```python
from build123d import *

# Parameters (mm, degrees)
SKETCH1_W           = 174
SKETCH1_H           = 148
SKETCH1_R           = 66
SKETCH1_R_2         = 2.15
BOSS_EXTRUDE1_DEPTH = 5
FILLET1_R           = 40


with BuildPart() as part:
    # Sketch1 → Boss-Extrude1 (new body)
    with BuildSketch(Plane(origin=(0, 0, 0), x_dir=(1, 0, 0), z_dir=(0, 1, 0))):
        Rectangle(SKETCH1_W, SKETCH1_H)
        with Locations(Location((0, 0, 0), (0, 0, 270))):
            Circle(SKETCH1_R, mode=Mode.SUBTRACT)
        with Locations(Location((75, 36, 0), (0, 0, 270))):
            Circle(SKETCH1_R_2, mode=Mode.SUBTRACT)
        with Locations(Location((75, 20, 0), (0, 0, 270))):
            Circle(SKETCH1_R_2, mode=Mode.SUBTRACT)
        with Locations(Location((75, -20, 0), (0, 0, 90))):
            Circle(SKETCH1_R_2, mode=Mode.SUBTRACT)
        with Locations(Location((75, -36, 0), (0, 0, 90))):
            Circle(SKETCH1_R_2, mode=Mode.SUBTRACT)
        with Locations(Location((-75, -36, 0), (0, 0, 270))):
            Circle(SKETCH1_R_2, mode=Mode.SUBTRACT)
        with Locations(Location((-75, -20, 0), (0, 0, 270))):
            Circle(SKETCH1_R_2, mode=Mode.SUBTRACT)
        with Locations(Location((-75, 20, 0), (0, 0, 90))):
            Circle(SKETCH1_R_2, mode=Mode.SUBTRACT)
        with Locations(Location((-75, 36, 0), (0, 0, 90))):
            Circle(SKETCH1_R_2, mode=Mode.SUBTRACT)
    extrude(amount=BOSS_EXTRUDE1_DEPTH)

    # Fillet1
    fillet1_edges = [part.edges().sort_by_distance(p)[0] for p in [
        (-87, 2.5, -74),
        (87, 2.5, -74),
        (87, 2.5, 74),
        (-87, 2.5, 74),
    ]]
    fillet(fillet1_edges, radius=FILLET1_R)


solid = part.part
```
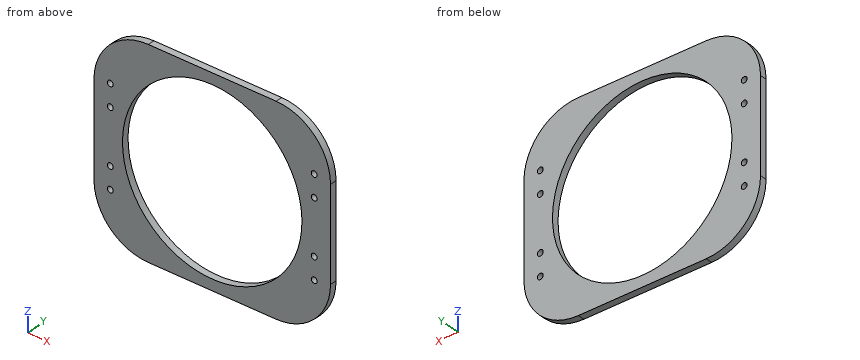
Design review of the part built by this model. Coordinates are the model's own, in mm. Coordinates: 2 decimals unless noted, no trailing zeros. Order: outer loops, then holes, each group sorted by start corner. A loop starts at its lowest first (then second) coordinate and runs counter-clockwise, first axis right, second up. Notation, with made-up numbers: M 30.5,31 L 46.5,31 A22 cw 46.5,64 Z; hole C 0,74.25 d10. An arc over 180 degrees is marked long. Answer as a JSON object with one key per item and string values. Group by question number.
1) For pin 1 (2.5 mm diameter, centred on x = 75, z = -36, fed in from +Y); pin 2 (3 mm diameter, centred on y = 0.5, z = -57.5, fed in from +X), all flat-tipped, find the tip position at first contact; note any pin that passes through.
2) Add section B-B, the plane y = 2.85. Count the separate pieces of the cut face and the enclosed holes in it, then the cut area to 3 significant figures.
3) Wall thickness on L1, parallel to X at y = 3.9, z = -20; L2, parallel to X at y = 2.1, z = 0; L3, parallel to X at y = 4, z = 36: over which ranges is each line inside the solid? List them lowest first.
4) Add section A-A, the plane z = 0. Write out the cut boundary in (x, y).
5) Add section C-C, the plane z = 20. Write out the cut boundary in (x, y).
6) Add section D-D, the plane x = 75. Write out the cut boundary in (y, z), then the cut area to 3 significant figures.
Computed values:
{
 "1": {"pin 1": "passes through", "pin 2": "stops at x = 80.41"},
 "2": {"separate pieces": "1", "enclosed holes": "9", "area": "10,600 mm^2"},
 "3": {"L1": "x = -87 to -77.15, -72.85 to -62.9, 62.9 to 72.85, 77.15 to 87", "L2": "x = -87 to -66, 66 to 87", "L3": "x = -86.95 to -77.15, -72.85 to -55.32, 55.32 to 72.85, 77.15 to 86.95"},
 "4": {"outline": "M -87,0 L -66,0 L -66,5 L -87,5 Z; M 66,0 L 87,0 L 87,5 L 66,5 Z"},
 "5": {"outline": "M -87,0 L -77.15,0 L -77.15,5 L -87,5 Z; M -72.85,0 L -62.9,0 L -62.9,5 L -72.85,5 Z; M 62.9,0 L 72.85,0 L 72.85,5 L 62.9,5 Z; M 77.15,0 L 87,0 L 87,5 L 77.15,5 Z"},
 "6": {"outline": "M 0,-62.57 L 5,-62.57 L 5,-38.15 L 0,-38.15 Z; M 0,-33.85 L 5,-33.85 L 5,-22.15 L 0,-22.15 Z; M 0,-17.85 L 5,-17.85 L 5,17.85 L 0,17.85 Z; M 0,22.15 L 5,22.15 L 5,33.85 L 0,33.85 Z; M 0,38.15 L 5,38.15 L 5,62.57 L 0,62.57 Z", "area": "540 mm^2"}
}
